Part model, mm, in its own coordinate system. Give positions to 0.01 mm unless a question says otherwise; leave off trailing zeros.
1. Slice it at A-A on y = 1.6. Give the number of separate pieces and of enclosed holes in the cut face, and give its area (3 significant figures).
2. Probe line 1 (Z direction, x = 220, y = 1.1); line 2 (Z direction, x = 279, y = 1.75). List the from-to ranges inside material, lowest first.
3. Drop flat-ended pins along their axis: pin 1 Ø3 at (x, z) = (220, 2.5) entering from +Y; pin 2 Ø1 at (y, z) = (1.5, 1) entering from +X. Give the stop position or say it passes through.
from build123d import *

# Parameters (mm, degrees)
SKETCH1_W           = 300
SKETCH1_H           = 5
BOSS_EXTRUDE1_DEPTH = 3
SKETCH2_R           = 1.6
CUT_EXTRUDE1_DEPTH  = 3


with BuildPart() as part:
    # Sketch1 → Boss-Extrude1 (new body)
    with BuildSketch(Plane(origin=(0, 0, 0), x_dir=(1, 0, 0), z_dir=(0, 1, 0))):
        with Locations((150, -2.5)):
            Rectangle(SKETCH1_W, SKETCH1_H)
    extrude(amount=BOSS_EXTRUDE1_DEPTH)

    # Sketch2 → Cut-Extrude1 (cut)
    with BuildSketch(Plane(origin=(0, 3, 0), x_dir=(1, 0, 0), z_dir=(0, 1, 0))):
        with Locations((0, -2.5)):
            Circle(SKETCH2_R)
        with Locations((20, -2.5)):
            Circle(SKETCH2_R)
        with Locations((40, -2.5)):
            Circle(SKETCH2_R)
        with Locations((60, -2.5)):
            Circle(SKETCH2_R)
        with Locations((80, -2.5)):
            Circle(SKETCH2_R)
        with Locations((100, -2.5)):
            Circle(SKETCH2_R)
        with Locations((120, -2.5)):
            Circle(SKETCH2_R)
        with Locations((140, -2.5)):
            Circle(SKETCH2_R)
        with Locations((160, -2.5)):
            Circle(SKETCH2_R)
        with Locations((180, -2.5)):
            Circle(SKETCH2_R)
        with Locations((200, -2.5)):
            Circle(SKETCH2_R)
        with Locations((220, -2.5)):
            Circle(SKETCH2_R)
        with Locations((240, -2.5)):
            Circle(SKETCH2_R)
        with Locations((260, -2.5)):
            Circle(SKETCH2_R)
        with Locations((280, -2.5)):
            Circle(SKETCH2_R)
        with Locations((300, -2.5)):
            Circle(SKETCH2_R)
        with Locations((320, -2.5)):
            Circle(SKETCH2_R)
        with Locations((340, -2.5)):
            Circle(SKETCH2_R)
        with Locations((360, -2.5)):
            Circle(SKETCH2_R)
        with Locations((380, -2.5)):
            Circle(SKETCH2_R)
        with Locations((400, -2.5)):
            Circle(SKETCH2_R)
        with Locations((420, -2.5)):
            Circle(SKETCH2_R)
        with Locations((440, -2.5)):
            Circle(SKETCH2_R)
        with Locations((460, -2.5)):
            Circle(SKETCH2_R)
        with Locations((480, -2.5)):
            Circle(SKETCH2_R)
        with Locations((500, -2.5)):
            Circle(SKETCH2_R)
        with Locations((520, -2.5)):
            Circle(SKETCH2_R)
        with Locations((540, -2.5)):
            Circle(SKETCH2_R)
        with Locations((560, -2.5)):
            Circle(SKETCH2_R)
        with Locations((580, -2.5)):
            Circle(SKETCH2_R)
        with Locations((600, -2.5)):
            Circle(SKETCH2_R)
        with Locations((620, -2.5)):
            Circle(SKETCH2_R)
        with Locations((640, -2.5)):
            Circle(SKETCH2_R)
        with Locations((660, -2.5)):
            Circle(SKETCH2_R)
        with Locations((680, -2.5)):
            Circle(SKETCH2_R)
        with Locations((700, -2.5)):
            Circle(SKETCH2_R)
        with Locations((720, -2.5)):
            Circle(SKETCH2_R)
        with Locations((740, -2.5)):
            Circle(SKETCH2_R)
        with Locations((760, -2.5)):
            Circle(SKETCH2_R)
        with Locations((780, -2.5)):
            Circle(SKETCH2_R)
        with Locations((800, -2.5)):
            Circle(SKETCH2_R)
        with Locations((820, -2.5)):
            Circle(SKETCH2_R)
        with Locations((840, -2.5)):
            Circle(SKETCH2_R)
        with Locations((860, -2.5)):
            Circle(SKETCH2_R)
        with Locations((880, -2.5)):
            Circle(SKETCH2_R)
        with Locations((900, -2.5)):
            Circle(SKETCH2_R)
        with Locations((920, -2.5)):
            Circle(SKETCH2_R)
        with Locations((940, -2.5)):
            Circle(SKETCH2_R)
        with Locations((960, -2.5)):
            Circle(SKETCH2_R)
        with Locations((980, -2.5)):
            Circle(SKETCH2_R)
        with Locations((1000, -2.5)):
            Circle(SKETCH2_R)
        with Locations((1020, -2.5)):
            Circle(SKETCH2_R)
        with Locations((1040, -2.5)):
            Circle(SKETCH2_R)
        with Locations((1060, -2.5)):
            Circle(SKETCH2_R)
        with Locations((1080, -2.5)):
            Circle(SKETCH2_R)
        with Locations((1100, -2.5)):
            Circle(SKETCH2_R)
        with Locations((1120, -2.5)):
            Circle(SKETCH2_R)
        with Locations((1140, -2.5)):
            Circle(SKETCH2_R)
        with Locations((1160, -2.5)):
            Circle(SKETCH2_R)
        with Locations((1180, -2.5)):
            Circle(SKETCH2_R)
        with Locations((1200, -2.5)):
            Circle(SKETCH2_R)
        with Locations((1220, -2.5)):
            Circle(SKETCH2_R)
        with Locations((1240, -2.5)):
            Circle(SKETCH2_R)
        with Locations((1260, -2.5)):
            Circle(SKETCH2_R)
        with Locations((1280, -2.5)):
            Circle(SKETCH2_R)
        with Locations((1300, -2.5)):
            Circle(SKETCH2_R)
        with Locations((1320, -2.5)):
            Circle(SKETCH2_R)
        with Locations((1340, -2.5)):
            Circle(SKETCH2_R)
        with Locations((1360, -2.5)):
            Circle(SKETCH2_R)
        with Locations((1380, -2.5)):
            Circle(SKETCH2_R)
        with Locations((1400, -2.5)):
            Circle(SKETCH2_R)
        with Locations((1420, -2.5)):
            Circle(SKETCH2_R)
        with Locations((1440, -2.5)):
            Circle(SKETCH2_R)
        with Locations((1460, -2.5)):
            Circle(SKETCH2_R)
        with Locations((1480, -2.5)):
            Circle(SKETCH2_R)
        with Locations((1500, -2.5)):
            Circle(SKETCH2_R)
        with Locations((1520, -2.5)):
            Circle(SKETCH2_R)
        with Locations((1540, -2.5)):
            Circle(SKETCH2_R)
        with Locations((1560, -2.5)):
            Circle(SKETCH2_R)
        with Locations((1580, -2.5)):
            Circle(SKETCH2_R)
        with Locations((1600, -2.5)):
            Circle(SKETCH2_R)
        with Locations((1620, -2.5)):
            Circle(SKETCH2_R)
        with Locations((1640, -2.5)):
            Circle(SKETCH2_R)
        with Locations((1660, -2.5)):
            Circle(SKETCH2_R)
        with Locations((1680, -2.5)):
            Circle(SKETCH2_R)
        with Locations((1700, -2.5)):
            Circle(SKETCH2_R)
        with Locations((1720, -2.5)):
            Circle(SKETCH2_R)
        with Locations((1740, -2.5)):
            Circle(SKETCH2_R)
        with Locations((1760, -2.5)):
            Circle(SKETCH2_R)
        with Locations((1780, -2.5)):
            Circle(SKETCH2_R)
        with Locations((1800, -2.5)):
            Circle(SKETCH2_R)
        with Locations((1820, -2.5)):
            Circle(SKETCH2_R)
        with Locations((1840, -2.5)):
            Circle(SKETCH2_R)
        with Locations((1860, -2.5)):
            Circle(SKETCH2_R)
        with Locations((1880, -2.5)):
            Circle(SKETCH2_R)
        with Locations((1900, -2.5)):
            Circle(SKETCH2_R)
        with Locations((1920, -2.5)):
            Circle(SKETCH2_R)
        with Locations((1940, -2.5)):
            Circle(SKETCH2_R)
        with Locations((1960, -2.5)):
            Circle(SKETCH2_R)
        with Locations((1980, -2.5)):
            Circle(SKETCH2_R)
    extrude(amount=-CUT_EXTRUDE1_DEPTH, mode=Mode.SUBTRACT)


solid = part.part
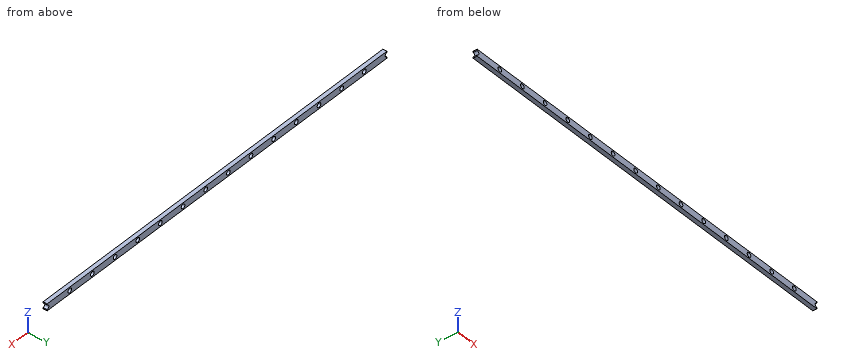
Data:
1. separate pieces: 1
1. enclosed holes: 14
1. area: 1,380 mm2
2. line 1: z = 0 to 0.9, 4.1 to 5
2. line 2: z = 0 to 1.25, 3.75 to 5
3. pin 1: passes through
3. pin 2: stops at x = 300
